from build123d import *

# Parameters (mm, degrees)
SKETCH1_R           = 2.54
BOSS_EXTRUDE2_DEPTH = 0.762


with BuildPart() as part:
    # Sketch1 → Boss-Extrude2 (new body)
    with BuildSketch(Plane.XY):
        with BuildLine():
            Line((-63.5, 88.9), (-63.5, 64.757547823))
            ThreePointArc((-63.5, 64.757547823), (-63.938471715, 62.438855663), (-65.193333333, 60.440377968))
            ThreePointArc((-65.193333333, 60.440377968), (0, -88.9), (65.193333333, 60.440377968))
            ThreePointArc((65.193333333, 60.440377968), (63.938471715, 62.438855663), (63.5, 64.757547823))
            Line((63.5, 64.757547823), (63.5, 88.9))
            ThreePointArc((63.5, 88.9), (0, 152.4), (-63.5, 88.9))
        make_face()
        with Locations((-71.490397082, -41.275)):
            Circle(SKETCH1_R, mode=Mode.SUBTRACT)
        with Locations((-71.490397082, 41.275)):
            Circle(SKETCH1_R, mode=Mode.SUBTRACT)
        with Locations((-57.15, 88.9)):
            Circle(SKETCH1_R, mode=Mode.SUBTRACT)
        with Locations((0, 146.05)):
            Circle(SKETCH1_R, mode=Mode.SUBTRACT)
        with Locations((57.15, 88.9)):
            Circle(SKETCH1_R, mode=Mode.SUBTRACT)
        with Locations((71.490397082, 41.275)):
            Circle(SKETCH1_R, mode=Mode.SUBTRACT)
        with Locations((71.490397082, -41.275)):
            Circle(SKETCH1_R, mode=Mode.SUBTRACT)
        with Locations((0, -82.55)):
            Circle(SKETCH1_R, mode=Mode.SUBTRACT)
        with BuildLine():
            Line((-53.975, 88.9), (-53.975, 64.757547823))
            ThreePointArc((-53.975, 64.757547823), (-55.071179287, 58.960817422), (-58.208333333, 53.964623186))
            ThreePointArc((-58.208333333, 53.964623186), (0, -79.375), (58.208333333, 53.964623186))
            ThreePointArc((58.208333333, 53.964623186), (55.071179287, 58.960817422), (53.975, 64.757547823))
            Line((53.975, 64.757547823), (53.975, 88.9))
            ThreePointArc((53.975, 88.9), (0, 142.875), (-53.975, 88.9))
        make_face(mode=Mode.SUBTRACT)
    extrude(amount=BOSS_EXTRUDE2_DEPTH)


solid = part.part
Verification items for the finished model (mm, model axes). A direction names the side the tool comes from. Round coordinates to 2 decimals unless told otherwise and drop trailing zeros. Order: outer loops, then holes, each group sorted by start corner. A loop starts at its lowest first (then second) coordinate and runs counter-clockwise, first axis right, second up.
1. Release check for a two-part mould opening along X. For faces 3 (the cylindrical face through (1.396, 152.385, 0.376)), 4 (the cylindrical face through (-0.55, -85.03, 0.38)), 5 (the flat face through (-60, 59, 0.762)) record: +X half, -X half, draft (parallel to the pull), parting line (faces both ways), or undercut.
Final values:
face 3: parting line
face 4: undercut
face 5: draft
2. Section check D-D on x = 47. Record the cut outline in (y, z).
Final values:
outline: (-75.46, 0) - (-63.96, 0) - (-63.96, 0.76) - (-75.46, 0.76) - close; (115.44, 0) - (131.6, 0) - (131.6, 0.76) - (115.44, 0.76) - close
3. Access from +Z, -Z, +X, -X, +Y, -Y to the whole of each face (thin tool, end or side, straight path). Record for faces 1 (the cylindrical face through (1.19, 142.86, 0.38)), 2 (the flat face through (-60, 59, 0)).
Final values:
face 1: +Z, -Z
face 2: -Z, +X, -X, +Y, -Y
4. Section check C-C on z = 0.6. State how many separate pieces and enclosed holes the cut face has, then the cut area to 3 significant figures.
Final values:
separate pieces: 1
enclosed holes: 9
area: 5,930 mm2
5. Thickness scan on L1, parallel to Y at x = 0, z = 0.35 (3 decimals); L2, parallel to X at y = 0, z = 0.5 (3 decimals); L3, parallel to Y at x = -57.15, z = 0.3. Record the ranges inside material, lowest first.
Final values:
L1: y = -88.9 to -85.09, -80.01 to -79.375, 142.875 to 143.51, 148.59 to 152.4
L2: x = -88.9 to -79.375, 79.375 to 88.9
L3: y = -68.1 to -55.08, 55.23 to 86.36, 91.44 to 116.58
6. Section check B-B on y = 0. Record the cut outline in (x, z) (3 decimals), then the cut area to 3 significant figures.
Final values:
outline: (-88.9, 0) - (-79.375, 0) - (-79.375, 0.762) - (-88.9, 0.762) - close; (79.375, 0) - (88.9, 0) - (88.9, 0.762) - (79.375, 0.762) - close
area: 14.5 mm2
7. Section check A-A on x = 0. Record the cut outline in (y, z) (3 decimals).
Final values:
outline: (-88.9, 0) - (-85.09, 0) - (-85.09, 0.762) - (-88.9, 0.762) - close; (-80.01, 0) - (-79.375, 0) - (-79.375, 0.762) - (-80.01, 0.762) - close; (142.875, 0) - (143.51, 0) - (143.51, 0.762) - (142.875, 0.762) - close; (148.59, 0) - (152.4, 0) - (152.4, 0.762) - (148.59, 0.762) - close
